Input: part model. Units: mm. Frame: model coordinates. Face numbers are marked on the shaded views. A direction names the side the tool comes from. Round coordinates to 2 decimals unless told otherwise and drop trailing zeros. Loops run counter-clockwise (first coordinate to the right, second up) from the corner with the lowest first, then second, coordinate; pieces in that order, holes last. Notation, with made-up numbers: M 68.5,-23.75 L 119.5,-23.75 A17 ccw 119.5,-1.75 Z; hole C 15,78.5 d8. An arc over 180 degrees is marked long. Use one line per item in the form item = value. Start each with the question number.
Q1. Section query C-C, the plane x = 6. Output: boundary loops of the cut face in (y, z).
Q2. Section query D-D, the plane x = 11.5. Output: boundary loops of the cut face in (y, z).
Q3. Section query A-A, the plane z = 0. Output: boundary loops of the cut face in (x, y), and give its area (3 significant figures).
Q4. First-contact query: P1, Ø2, axis at y = 0, z = -4, coming from the -X side; P2, Ø1.5, axis at x = 4.5, y = 2, coming from the +Z side; P3, Ø6, axis at x = 8, z = 1.5, coming from the -Y side; P4, Ø5, axis at x = 10, z = -2.5, coming from the -Y side. Flat tips, straight axial feed; report the tip coordinate or a pass-through.
Q5. Access query for the marked faces 1 and 2. Directions: +Z, -Z, +X, -X, +Y, -Y. A direction counts if a zero-diameter tool reaches every point of the face in a straight line with its end or side. Return the directions, or none.
Q6. Ray query, line 1 along X through (y, z) = (-2.75, -1.25); line 2 along Y through (x, z) = (7.25, -4.25); line 3 along Y through (x, z) = (3.25, 3). Return the intervals inside material, ascending.
```python
from build123d import *

# Parameters (mm, degrees)
FILETE1_R = 0.5
FILETE2_R = 0.5


with BuildPart() as part:
    # Esboço1 → Revolução1 (revolve)
    with BuildSketch(Plane.XY):
        Polygon((0, 0), (0, 3), (7.5, 5.3), (7.5, 5), (12.5, 5), (12.5, 0), align=None)
    revolve(axis=Axis((12.5, 0, 0), (-1, 0, 0)))

    # Filete1
    filete1_edges = [part.edges().sort_by_distance(p)[0] for p in [
        (12.5, -5, 0),
    ]]
    fillet(filete1_edges, radius=FILETE1_R)

    # Filete2
    filete2_edges = [part.edges().sort_by_distance(p)[0] for p in [
        (0, -3, 0),
    ]]
    fillet(filete2_edges, radius=FILETE2_R)


solid = part.part
```
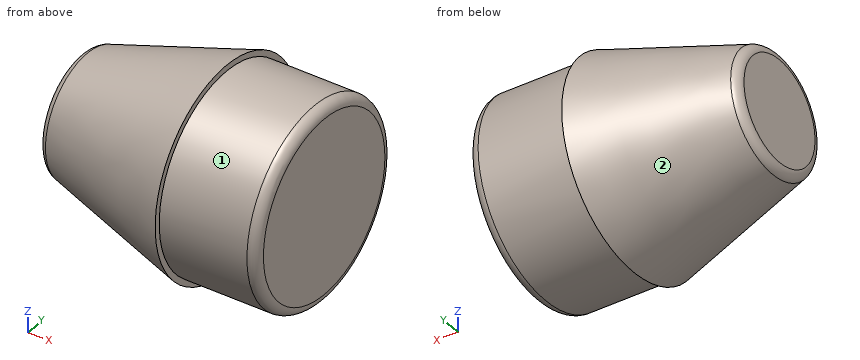
Results found:
q1.outline = C 0,0 d9.68
q2.outline = C 0,0 d10
q3.outline = M 0,-2.63 A0.5 ccw 0.35,-3.11 L 7.5,-5.3 L 7.5,-5 L 12,-5 A0.5 ccw 12.5,-4.5 L 12.5,4.5 A0.5 ccw 12,5 L 7.5,5 L 7.5,5.3 L 0.35,3.11 A0.5 ccw 0,2.63 Z
q3.area = 112 mm²
q4.P1 = 0.16
q4.P2 = 4.3
q4.P3 = -5.3
q4.P4 = -5
q5.face_1 = +X
q5.face_2 = -X
q6.line_1 = 0.19 to 12.5
q6.line_2 = -3.04 to 3.04
q6.line_3 = -2.64 to 2.64
